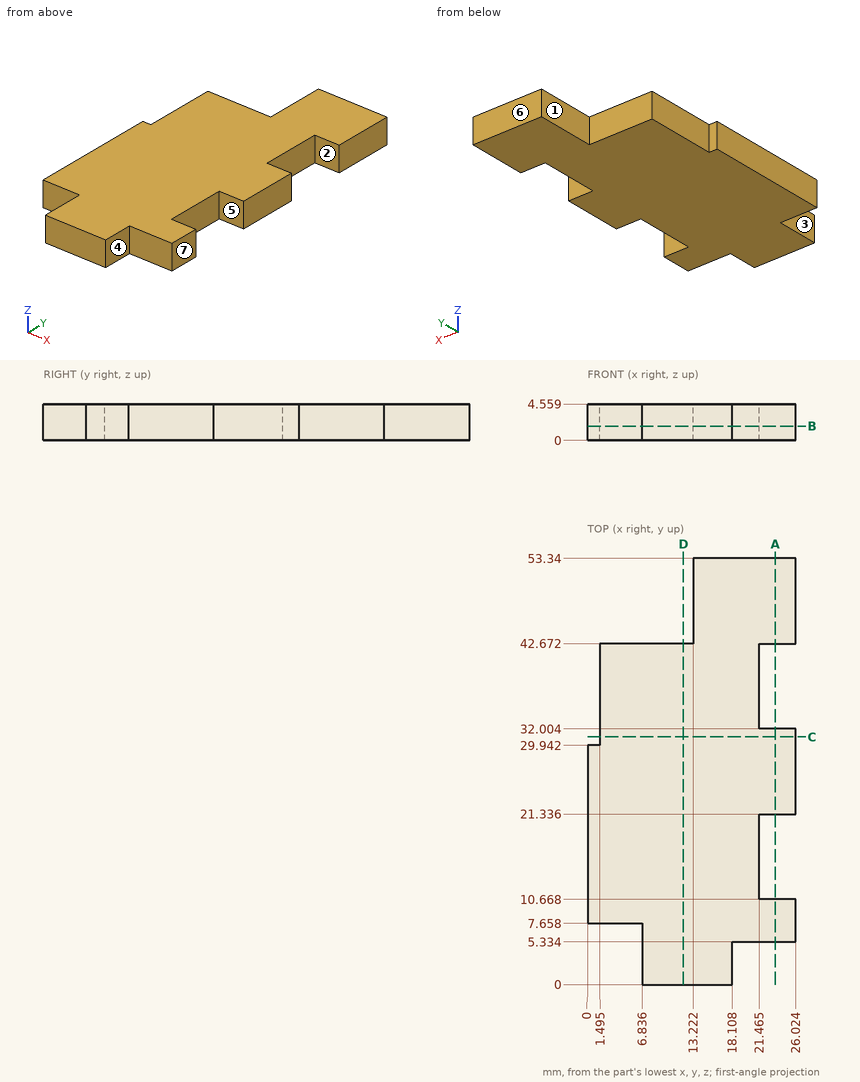
Answer from the drawing. Dimensions are ordinates in mm from the lowest x, y and z of the part. A direction names the side the tool comes from. Give positions to 0.01 mm unless a question says otherwise; leave off trailing zeros. Write each loop counter-clockwise with the first axis right and the second up, starting at its lowest first coordinate (ties: lowest second). Pieces come first, ordered by that corner, then holes.
1) Section A-A (x = 23.5) is taken. Write down the section's boundary in (y, z), and give its area (3 significant figures).
2) A tool of negligible diameter and unlimited length cuts with its end or side. For the marked faces 1, 2, 3 and 4, from which of +Z, -Z, +X, -X, +Y, -Y can it reach the whole face along a straight path? Write none if from no direction.
3) Section B-B (z = 1.8) is taken. Write down the section's boundary in (x, y) (1 decimal), and give its area (3 significant figures).
4) Section C-C (y = 31) is taken. Write down the section's boundary in (x, z) (1 decimal), and give its area (3 significant figures).
5) Given P1, Ø1, axis at y = 40, z = 1.5, coming from the +X side (1 decimal); P2, Ø1.4, axis at y = 3.5, z = 3, coming from the +X side; P3, Ø1.4, axis at x = 2.5, z = 3.5, coming from the -Y side, each flat-ended and moving along its own axis, determine where each tip first touches the part or whether it passes through.
6) For a pull along Y with two mould halves and no side action, classify the marked faces 5, 6 and 7 as pulls with the +Y half, pulls with the -Y half, needs draft (parallel to the pull), parting line crosses it, or undercut.
7) Find the intervals of material crossed by L1, parallel to Y at x = 21.75, z = 1.75; L2, parallel to X at y = 35, z = 2.4 (1 decimal); L3, parallel to Y at x = 19, z = 1.9, in increasing order.
8) Section D-D (x = 12) is taken. Write down the section's boundary in (y, z).
Response:
1. outline: (5.33, 0) - (10.67, 0) - (10.67, 4.56) - (5.33, 4.56) - close; (21.34, 0) - (32, 0) - (32, 4.56) - (21.34, 4.56) - close; (42.67, 0) - (53.34, 0) - (53.34, 4.56) - (42.67, 4.56) - close
1. area: 122 mm2
2. face 1: +Z, -Z, -X, +Y
2. face 2: +Z, -Z, +X
2. face 3: +Z, -Z, -X, -Y
2. face 4: +Z, -Z, +X, -Y
3. outline: (0, 7.7) - (6.8, 7.7) - (6.8, 0) - (18.1, 0) - (18.1, 5.3) - (26, 5.3) - (26, 10.7) - (21.5, 10.7) - (21.5, 21.3) - (26, 21.3) - (26, 32) - (21.5, 32) - (21.5, 42.7) - (26, 42.7) - (26, 53.3) - (13.2, 53.3) - (13.2, 42.7) - (1.5, 42.7) - (1.5, 29.9) - (0, 29.9) - close
3. area: 1,040 mm2
4. outline: (1.5, 0) - (26, 0) - (26, 4.6) - (1.5, 4.6) - close
4. area: 112 mm2
5. P1: stops at x = 21.5
5. P2: stops at x = 18.11
5. P3: stops at y = 7.66
6. face 5: undercut
6. face 6: pulls with the +Y half
6. face 7: needs draft
7. L1: y = 5.33 to 10.67, 21.34 to 32, 42.67 to 53.34
7. L2: x = 1.5 to 21.5
7. L3: y = 5.33 to 53.34
8. outline: (0, 0) - (42.67, 0) - (42.67, 4.56) - (0, 4.56) - close
